from build123d import *

# Parameters (mm, degrees)
FILLET1_R     = 0.2
CHAMFER1_SIZE = 0.5


with BuildPart() as part:
    # Sketch1 → Revolve1 (revolve)
    with BuildSketch(Plane.XY, mode=Mode.PRIVATE) as revolve1_sk:
        Polygon((0, 0), (5, 0), (5, 65.35), (4, 65.35), (4, 122), (0, 122), align=None)
    revolve(revolve1_sk.sketch.rotate(Axis((0, 7.476190476, 0), (0, -1, 0)), 90), axis=Axis((0, 7.476190476, 0), (0, -1, 0)))

    # Sketch4 → M4 Tapped Hole1 (revolve, cut)
    with BuildSketch(Plane(origin=(0, 0, 0), x_dir=(0, 0, -1), z_dir=(1, 0, 0))):
        Polygon((0, 0), (0, 12.991420021), (1.65, 12), (1.65, 0), align=None)
    m4_tapped_hole1 = revolve(axis=Axis((0, -6.35, 0), (0, 1, 0)), mode=Mode.SUBTRACT)

    # Mirror1: M4 Tapped Hole1 across plane
    add(m4_tapped_hole1.mirror(Plane(origin=(0, 61, 0), x_dir=(0, 0, 1), z_dir=(0, -1, 0))), mode=Mode.SUBTRACT)

    # Fillet1
    fillet1_edges = [part.edges().sort_by_distance(p)[0] for p in [
        (0, 65.35, -4),
    ]]
    fillet(fillet1_edges, radius=FILLET1_R)

    # Chamfer1
    chamfer1_edges = [part.edges().sort_by_distance(p)[0] for p in [
        (0, 122, -4),
        (0, 65.35, -5),
        (0, 0, -5),
    ]]
    chamfer(chamfer1_edges, length=CHAMFER1_SIZE)


solid = part.part
The listing builds one solid part. Answer for the finished solid, in the listing's coordinates (mm). A direction names the side the tool comes from. Give positions to 0.01 mm unless a question says otherwise; leave off trailing zeros. Order: outer loops, then holes, each group sorted by start corner. A loop starts at its lowest first (then second) coordinate and runs counter-clockwise, first axis right, second up. Notation, with made-up numbers: (21.5, -18.75) - (48.5, -18.75) arc R33 cw to (48.5, 19.25) - close; hole circle Ø3 at (-10.75, 43.25). An arc over 180 degrees is marked (long way). One line per item, written item: value. Start each with the question number.
1) A cutting plane is placed at A-A on y = 81.5. Give the vertices of the cut face in (x, z), then the cut area to 3 significant figures.
2) Find the intervals of material crossed by L1, parallel to X at y = 5.5, z = 0; L2, parallel to X at y = 113, z = 0; L3, parallel to X at y = 93, z = -2.25, in increasing order.
3) A tool of negligible diameter and unlimited length cuts with its end or side. For faces 1 (the face through (-1.115, 5.916, 1.216)), 2 (the face through (2, 122, 1)), 3 (the face through (-1.115, 116.084, 1.216)), from which of +Z, -Z, +X, -X, +Y, -Y can it reach the whole face along a straight path? Write none if from no direction.
4) A cutting plane is placed at B-B on y = 47.5. Give the vertices of the cut face in (x, z), then the cut area to 3 significant figures.
5) Given pin 1 Ø6 at (y, z) = (87.5, -3.5) entering from -X; pin 2 Ø6 at (y, z) = (84.5, -4) entering from -X; pin 3 Ø1.5 at (x, y) = (-1, 96.5) entering from +Z, each flat-ended and moving along its own axis, determine where each tip first touches the part or whether it passes through.
6) The mould has two halves that part along X. Classify faces 4 (the face through (0.3, 12.8, 0.1)), 5 (the face through (2, 0, 0)), 6 (the face through (0, 33, -5)): released by +X, released by -X, zero draft, split by the parting line, or undercut.
Answer sheet:
1. outline: circle Ø8 at (0, 0)
1. area: 50.3 mm2
2. L1: x = -5 to -1.65, 1.65 to 5
2. L2: x = -4 to -1.65, 1.65 to 4
2. L3: x = -3.31 to 3.31
3. face 1: -Y
3. face 2: +Z, -Z, +X, -X, +Y
3. face 3: +Y
4. outline: circle Ø10 at (0, 0)
4. area: 78.5 mm2
5. pin 1: stops at x = -3.97
5. pin 2: stops at x = -3.87
5. pin 3: stops at z = 3.99
6. face 4: undercut
6. face 5: zero draft
6. face 6: split by the parting line
